```python
from build123d import *

# Parameters (mm, degrees)
EXTRUDE_1_DEPTH     = 7
CUT_EXTRUDE_1_DEPTH = 49.546658999
F_4_0MM_2_OUTLINE_R = 2
F_4_0MM_2_DEPTH     = 7
SKETCH_6_R          = 20.5
CUT_EXTRUDE_2_DEPTH = 2


# Read off the part's stored shape, not the designer's step: Ø4.0mm 暗销孔2
with BuildPart() as part:
    # 草图2 → 凸台-拉伸1 (new body)
    with BuildSketch(Plane.XY):
        with BuildLine():
            Line((-36.1, 27.91), (36.1, 27.91))
            ThreePointArc((36.1, 27.91), (38.221320344, 27.031320344), (39.1, 24.91))
            Line((39.1, 24.91), (39.1, -24.91))
            ThreePointArc((39.1, -24.91), (38.221320344, -27.031320344), (36.1, -27.91))
            Line((36.1, -27.91), (-36.1, -27.91))
            ThreePointArc((-36.1, -27.91), (-38.221320344, -27.031320344), (-39.1, -24.91))
            Line((-39.1, -24.91), (-39.1, 24.91))
            ThreePointArc((-39.1, 24.91), (-38.221320344, 27.031320344), (-36.1, 27.91))
        make_face()
    extrude(amount=EXTRUDE_1_DEPTH)

    # 草图1 → 切除-拉伸1 (cut, through all)
    with BuildSketch(Plane.XY):
        with BuildLine():
            Line((-31.5, 18.05), (-31.5, 21))
            Line((-31.5, 21), (-28.55, 21))
            ThreePointArc((-28.55, 21), (-33.585965005, 23.085965005), (-31.5, 18.05))
        make_face()
        with BuildLine():
            Line((-28.55, 21), (-31.5, 21))
            Line((-31.5, 21), (-31.5, 18.05))
            ThreePointArc((-31.5, 18.05), (-29.414034995, 18.914034995), (-28.55, 21))
        make_face()
        with BuildLine():
            ThreePointArc((34.45, 21), (31.5, 23.95), (28.55, 21))
            Line((28.55, 21), (31.5, 21))
            Line((31.5, 21), (31.5, 18.05))
            ThreePointArc((31.5, 18.05), (33.585965005, 18.914034995), (34.45, 21))
        make_face()
        with BuildLine():
            Line((31.5, 21), (28.55, 21))
            ThreePointArc((28.55, 21), (29.414034995, 18.914034995), (31.5, 18.05))
            Line((31.5, 18.05), (31.5, 21))
        make_face()
        with BuildLine():
            ThreePointArc((-28.55, -21), (-29.414034995, -18.914034995), (-31.5, -18.05))
            Line((-31.5, -18.05), (-31.5, -21))
            Line((-31.5, -21), (-28.55, -21))
        make_face()
        with BuildLine():
            Line((-31.5, -21), (-31.5, -18.05))
            ThreePointArc((-31.5, -18.05), (-33.585965005, -23.085965005), (-28.55, -21))
            Line((-28.55, -21), (-31.5, -21))
        make_face()
        with BuildLine():
            ThreePointArc((34.45, -21), (33.585965005, -18.914034995), (31.5, -18.05))
            Line((31.5, -18.05), (31.5, -21))
            Line((31.5, -21), (28.55, -21))
            ThreePointArc((28.55, -21), (31.5, -23.95), (34.45, -21))
        make_face()
        with BuildLine():
            Line((31.5, -21), (31.5, -18.05))
            ThreePointArc((31.5, -18.05), (29.414034995, -18.914034995), (28.55, -21))
            Line((28.55, -21), (31.5, -21))
        make_face()
    extrude(amount=CUT_EXTRUDE_1_DEPTH, mode=Mode.SUBTRACT)

    # Ø4.0mm 暗销孔2 outline → Ø4.0mm 暗销孔2 (cut)
    with BuildSketch(Plane.XY):
        with Locations((8.980256121, -8.980256121)):
            Circle(F_4_0MM_2_OUTLINE_R)
        with Locations((-8.980256121, -8.980256121)):
            Circle(F_4_0MM_2_OUTLINE_R)
        with Locations((-8.980256121, 8.980256121)):
            Circle(F_4_0MM_2_OUTLINE_R)
        with Locations((8.980256121, 8.980256121)):
            Circle(F_4_0MM_2_OUTLINE_R)
    extrude(amount=F_4_0MM_2_DEPTH, mode=Mode.SUBTRACT)

    # 草图6 → 切除-拉伸2 (cut)
    with BuildSketch(Plane(origin=(0, 0, 0), x_dir=(-1, 0, 0), z_dir=(0, 0, -1))):
        Circle(SKETCH_6_R)
    extrude(amount=-CUT_EXTRUDE_2_DEPTH, mode=Mode.SUBTRACT)


solid = part.part
```
The model under review builds one solid part; all positions refer to its coordinate system, in mm. A direction names the side the tool comes from. Coordinates: 2 decimals unless noted, no trailing zeros. Order: outer loops, then holes, each group sorted by start corner. A loop starts at its lowest first (then second) coordinate and runs counter-clockwise, first axis right, second up. Notation, with made-up numbers: (52, -3) -> (88, -3) arc R12 cw to (88, 17) -> close; hole circle Ø5 at (-37, 1.5). An arc over 180 degrees is marked (long way). Answer in a Markdown table with one row per item. Add a question column.
Item 1: We need section C-C on x = -10. Write out the cut boundary in (y, z), plus the area to 3 significant figures.
Item 2: Clearance check with flat-ended pins moving along their axes: pin 1 (2.5 mm diameter, centred on x = 8.98, y = -8.98, fed in from -Z); pin 2 (6.5 mm diameter, centred on x = -8.98, y = 8.98, fed in from -Z). State where each tip first meets the part, or that it passes through.
Item 3: To check wall thickness, follow probe 1 along X at (y, z) = (-21, 2); probe 2 along Y at (x, z) = (-31.5, 3.5); probe 3 along X at (y, z) = (-23, 1). State the ranges of each line that lie inside material, in increasing order.
Item 4: Machinability: for faces 4 (the cylindrical face through (-7.073, 9.581, 4.465)), 5 (the cylindrical face through (4.444, -20.013, 0.986)), which of the approach directions +Z, -Z, +X, -X, +Y, -Y give a long, thin tool a straight path to every point of the face, cutting with its end or side? Answer none if there is none.
Item 5: We need section B-B on x = 0. Write out the cut boundary in (y, z).
Item 6: We need section D-D on y = 19.5. Write out the cut boundary in (x, z).
Item 7: We need section A-A on z = 1. Write out the cut boundary in (x, y).
Item 8: Mouldability with a two-part tool opening along Y and no side actions: class faces 1 (the cylindrical face through (-38.24, 27.01, 3.45)), 2 (the flat face through (1, -27.91, 3)), 3 (the flat face through (0, 0, 2)) as +Y half, -Y half, draft (parallel to the pull), parting line (faces both ways), or undercut.
Final values:
| question | item | result |
|---|---|---|
| 1 | outline | (-27.91, 0) -> (-17.9, 0) -> (-17.9, 2) -> (-10.7, 2) -> (-10.7, 7) -> (-27.91, 7) -> close; (-7.26, 2) -> (7.26, 2) -> (7.26, 7) -> (-7.26, 7) -> close; (10.7, 2) -> (17.9, 2) -> (17.9, 0) -> (27.91, 0) -> (27.91, 7) -> (10.7, 7) -> close |
| 1 | area | 285 mm2 |
| 2 | pin 1 | passes through |
| 2 | pin 2 | stops at z = 2 |
| 3 | probe 1 | x = -39.1 to -34.45, -28.55 to 28.55, 34.45 to 39.1 |
| 3 | probe 2 | y = -27.91 to -23.95, -18.05 to 18.05, 23.95 to 27.91 |
| 3 | probe 3 | x = -39.1 to -33.67, -29.33 to 29.33, 33.67 to 39.1 |
| 4 | face 4 | +Z, -Z |
| 4 | face 5 | -Z |
| 5 | outline | (-27.91, 0) -> (-20.5, 0) -> (-20.5, 2) -> (20.5, 2) -> (20.5, 0) -> (27.91, 0) -> (27.91, 7) -> (-27.91, 7) -> close |
| 6 | outline | (-39.1, 0) -> (-34.04, 0) -> (-34.04, 7) -> (-39.1, 7) -> close; (-28.96, 0) -> (-6.32, 0) -> (-6.32, 2) -> (6.32, 2) -> (6.32, 0) -> (28.96, 0) -> (28.96, 7) -> (-28.96, 7) -> close; (34.04, 0) -> (39.1, 0) -> (39.1, 7) -> (34.04, 7) -> close |
| 7 | outline | (-39.1, -24.91) arc R3 ccw to (-36.1, -27.91) -> (36.1, -27.91) arc R3 ccw to (39.1, -24.91) -> (39.1, 24.91) arc R3 ccw to (36.1, 27.91) -> (-36.1, 27.91) arc R3 ccw to (-39.1, 24.91) -> close; hole circle Ø5.9 at (-31.5, -21); hole circle Ø5.9 at (-31.5, 21); hole circle Ø41 at (0, 0); hole circle Ø5.9 at (31.5, -21); hole circle Ø5.9 at (31.5, 21) |
| 8 | face 1 | +Y half |
| 8 | face 2 | -Y half |
| 8 | face 3 | undercut |
